The figure shows three views and two pictorial views of one solid part (mm, origin at its lowest corner). Answer the questions. Round coordinates to 2 decimals unless told otherwise and drop trailing zeros. Loops run counter-clockwise (first coordinate to the right, second up) from the corner with the lowest first, then second, coordinate; pieces in that order, holes last. Notation, with made-up numbers: (40, 81) -> (85, 81) arc R21 cw to (85, 109) -> close; hole circle Ø9 at (81.5, 78.5). An arc over 180 degrees is marked (long way). Use a Markdown table: item, result. Add a question column.
Q1. Given pin 1 Ø8 at (x, z) = (20.5, 11) entering from +Y, flat-ended and moving along its own axis, determine where the tip first touches the part or whether it passes through.
Q2. Consider line 1 (X direction, y = 1.35, z = 20); line 2 (Z direction, x = 6.25, y = 0.35); line 3 (X direction, y = 0.2, z = 5.75). Determine where each line is inside the solid, lowest interval first.
Q3. Section C-C on x = 24 is taken. Give the vertices of the cut face in (y, z).
Q4. Section B-B on x = 11.75 is taken. Give the vertices of the cut face in (y, z).
Q5. Section A-A on y = 0.35 is taken. Give the vertices of the cut face in (x, z), then the cut area to 3 significant figures.
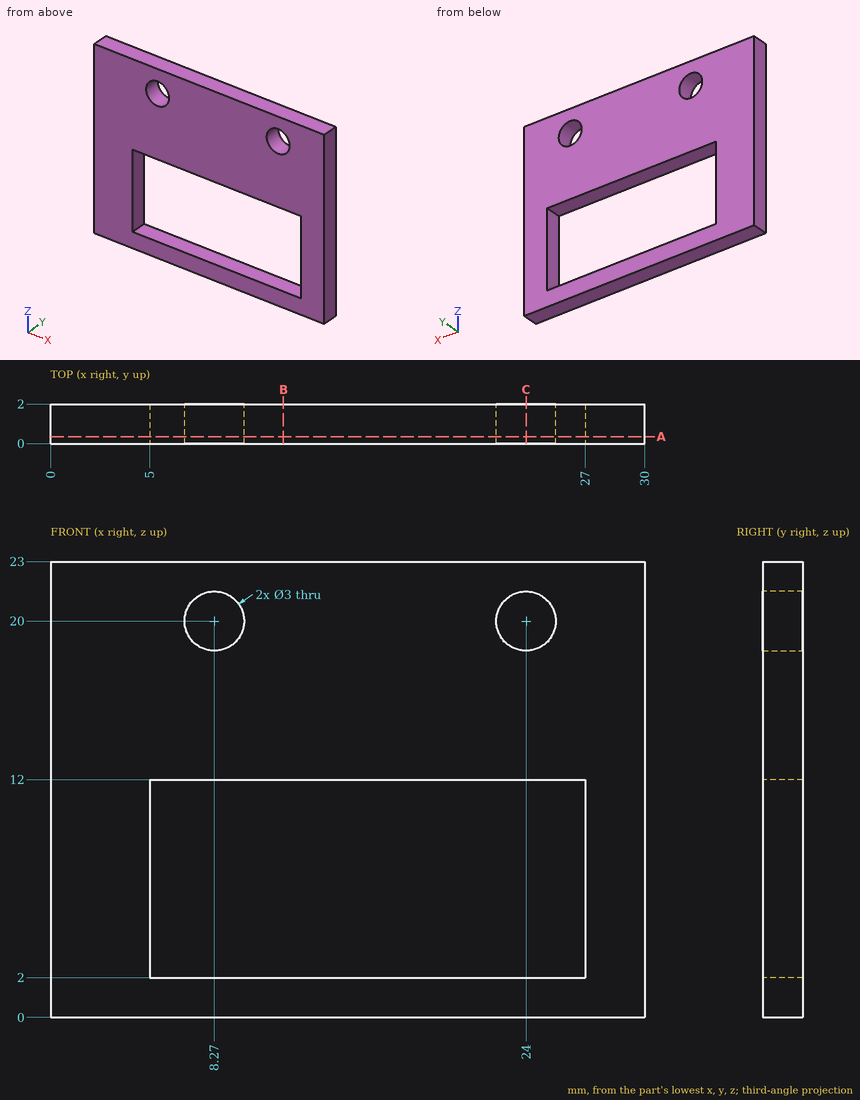
Checked values:
| question | item | result |
|---|---|---|
| 1 | pin 1 | stops at y = 2 |
| 2 | line 1 | x = 0 to 6.77, 9.77 to 22.5, 25.5 to 30 |
| 2 | line 2 | z = 0 to 2, 12 to 23 |
| 2 | line 3 | x = 0 to 5, 27 to 30 |
| 3 | outline | (0, 0) -> (2, 0) -> (2, 2) -> (0, 2) -> close; (0, 12) -> (2, 12) -> (2, 18.5) -> (0, 18.5) -> close; (0, 21.5) -> (2, 21.5) -> (2, 23) -> (0, 23) -> close |
| 4 | outline | (0, 0) -> (2, 0) -> (2, 2) -> (0, 2) -> close; (0, 12) -> (2, 12) -> (2, 23) -> (0, 23) -> close |
| 5 | outline | (0, 0) -> (30, 0) -> (30, 23) -> (0, 23) -> close; hole (5, 2) -> (27, 2) -> (27, 12) -> (5, 12) -> close; hole circle Ø3 at (8.27, 20); hole circle Ø3 at (24, 20) |
| 5 | area | 456 mm2 |
